The listing builds one solid part. Answer for the finished solid, in the listing's coordinates (mm). Coordinates: 2 decimals unless noted, no trailing zeros. Write each loop counter-clockwise with the first axis right and the second up, starting at its lowest first coordinate (ties: lowest second). Pieces come first, ordered by that corner, then holes.
(1) Straight lines are drawn through the part: line 1 (Y direction, x = 0, z = 22.15); line 2 (Y direction, x = 0, z = 12); line 3 (X direction, y = -4.5, z = 5.25). For each, find the intervals that lie inside material, in ascending order.
(2) The part is cut by section D-D on z = 16. Determine the outline of the cut face in (x, y).
(3) The part is cut by section A-A on y = 0. Determine the outline of the cut face in (x, z).
(4) The part is cut by section C-C on y = -184. Determine the outline of the cut face in (x, z), plus the area to 3 significant figures.
(5) The part is cut by section B-B on x = 0. Determine the outline of the cut face in (y, z).
(6) Given P1, Ø12, axis at x = 102, z = 10, coming from the -Y side; P2, Ø1, axis at x = 126.5, z = 3, coming from the +Y side; P3, Ø4, axis at y = 136, z = 4.5, coming from the -X side, each flat-ended and moving along its own axis, determine where each tip first touches the part or whether it passes through.
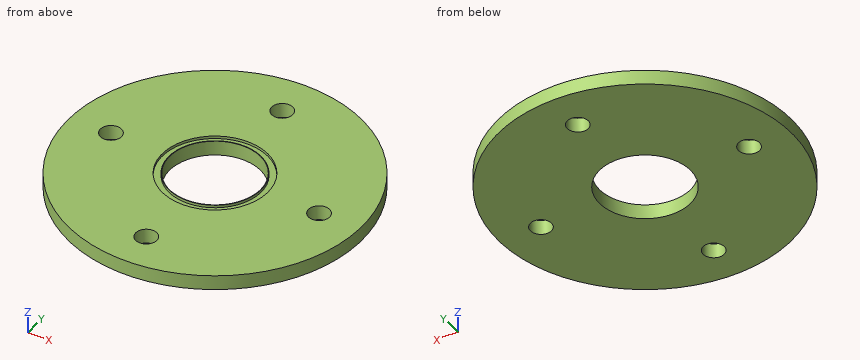
Autodesk Inventor part; units mm, degrees
ref_plane "YZ Plane" through (0, 0, 0) normal (1, 0, 0) x (0, 1, 0)
ref_plane "XZ Plane" through (0, 0, 0) normal (0, 1, 0) x (-1, 0, 0)
ref_plane "XY Plane" through (0, 0, 0) normal (0, 0, 1) x (1, 0, 0)
sketch "Szkic1" plane through (0, 0, 0) normal (0, 0, 1) x (1, 0, 0)
  circle A0 centre (0, 0) radius 250
  dimension "d0" = 500
extrude "Wyciągnięcie proste1" add sketch "Szkic1" along normal blind 25
sketch "Szkic2" plane through (0, 0, 25) normal (0, 0, 1) x (1, 0, 0)
  circle A0 centre (0, 180) radius 18
  circle A1 centre (180, 0) radius 18
  circle A2 centre (0, -184) radius 18
  circle A3 centre (-180, 0) radius 18
  point P0 (0, 0)
  dimension "d3" = 36
  dimension "d4" = 36
  dimension "d5" = 36
  dimension "d6" = 36
extrude "Wyciągnięcie proste2" cut sketch "Szkic2" against normal blind 25
thread "Gwint1"
thread "Gwint2"
thread "Gwint3"
thread "Gwint4"
sketch "Szkic3" plane through (0, 0, 25) normal (0, 0, 1) x (1, 0, 0)
  circle A0 centre (0, 0) radius 85
  dimension "d17" = 170
extrude "Wyciągnięcie proste3" cut sketch "Szkic3" against normal blind 200
sketch "Szkic4" plane through (0, 0, 25) normal (0, 0, 1) x (1, 0, 0)
  circle A0 centre (0, 0) radius 77.5
  dimension "d20" = 155
sketch "Szkic5" plane through (0, 0, 25) normal (0, 0, 1) x (1, 0, 0)
  circle A0 centre (0, 0) radius 85
  dimension "d21" = 170
extrude "Wyciągnięcie proste4" add sketch "Szkic5" against normal blind 25
extrude "Wyciągnięcie proste5" cut sketch "Szkic4" against normal blind 25
sketch "Szkic6" plane through (0, 0, 25) normal (0, 0, 1) x (1, 0, 0)
  circle A0 centre (0, 0) radius 82
  circle A1 centre (0, 0) radius 87
  dimension "d26" = 164
  dimension "d27" = 174
extrude "Wyciągnięcie proste6" cut sketch "Szkic6" against normal blind 4.5
sketch "Szkic7" plane through (0, 0, 25) normal (0, 0, 1) x (1, 0, 0)
  circle A0 centre (0, 0) radius 79.5
  circle A1 centre (0, 0) radius 84.5
  dimension "d30" = 159
  dimension "d31" = 169
extrude "Wyciągnięcie proste7" cut sketch "Szkic7" against normal blind 4.5
sketch "Szkic8" plane through (0, 0, 25) normal (0, 0, 1) x (1, 0, 0)
  circle A0 centre (0, 0) radius 78.5
  circle A1 centre (0, 0) radius 90
  dimension "d34" = 157
  dimension "d36" = 180
extrude "Wyciągnięcie proste8" cut sketch "Szkic8" against normal blind 4.5
properties part number "pięćśetka"
Model answer:
1. line 1: y = -250 to -202, -166 to -90, -78.5 to -77.5, 77.5 to 78.5, 90 to 162, 198 to 250
1. line 2: y = -250 to -202, -166 to -77.5, 77.5 to 162, 198 to 250
1. line 3: x = -249.96 to -197.43, -162.57 to -77.37, 77.37 to 162.57, 197.43 to 249.96
2. outline: circle Ø500 at (0, 0); hole circle Ø36 at (-180, 0); hole circle Ø155 at (0, 0); hole circle Ø36 at (0, -184); hole circle Ø36 at (0, 180); hole circle Ø36 at (180, 0)
3. outline: (-250, 0) - (-198, 0) - (-198, 25) - (-250, 25) - close; (-162, 0) - (-77.5, 0) - (-77.5, 25) - (-78.5, 25) - (-78.5, 20.5) - (-90, 20.5) - (-90, 25) - (-162, 25) - close; (77.5, 0) - (162, 0) - (162, 25) - (90, 25) - (90, 20.5) - (78.5, 20.5) - (78.5, 25) - (77.5, 25) - close; (198, 0) - (250, 0) - (250, 25) - (198, 25) - close
4. outline: (-169.25, 0) - (-18, 0) - (-18, 25) - (-169.25, 25) - close; (18, 0) - (169.25, 0) - (169.25, 25) - (18, 25) - close
4. area: 7,560 mm2
5. outline: (-250, 0) - (-202, 0) - (-202, 25) - (-250, 25) - close; (-166, 0) - (-77.5, 0) - (-77.5, 25) - (-78.5, 25) - (-78.5, 20.5) - (-90, 20.5) - (-90, 25) - (-166, 25) - close; (77.5, 0) - (162, 0) - (162, 25) - (90, 25) - (90, 20.5) - (78.5, 20.5) - (78.5, 25) - (77.5, 25) - close; (198, 0) - (250, 0) - (250, 25) - (198, 25) - close
6. P1: stops at y = -230.83
6. P2: stops at y = 215.93
6. P3: stops at x = -211.05
